Here's how the part is built. I have some questions about the finished solid (model axes, mm). Give positions to 0.01 mm unless a question says otherwise; leave off trailing zeros. Write each loop counter-clockwise with the first axis right and the second up, starting at its lowest first coordinate (ties: lowest second). Pieces come first, ordered by that corner, then holes. Notation, with made-up numbers: (58.25, 14.5) - (86.25, 14.5) arc R10 ccw to (86.25, 33.5) - close; hole circle Ø7 at (-11, -24). An arc over 180 degrees is marked (long way). Write each question's results on one line, items separated by ' | '. Start each with the question number.
Item 1: Suppose I cut it at B-B on z = -24. List the corners of the cut face in (x, y) for me.
Item 2: We'd pull the mould along Z, two halves only. Please class faces 1 (the flat face through (13.496, 1.503, 10.13)), 2 (the flat face through (12.676, 1.503, 60.654)), 3 (the flat face through (2, 3.048, 14)), 4 (the cylindrical face through (-15.875, 1.503, 34.414)): +Z half, -Z half, draft (parallel to the pull), parting line (faces both ways), or undercut.
Item 3: Please list where these lines run through material, in increasing order: line 1 along Z through (x, y) = (-6, 1.7); line 2 along Z through (x, y) = (38, 0.8); line 3 along X through (y, z) = (2.15, -29.5).
Item 4: Will these pins go through, and if not, where does the flat tip stop? P1, Ø1.5, axis at x = 18, y = 1.5, coming from the -Z side; P2, Ø1.5, axis at x = -8.5, y = 2.5, coming from the -Z side; P3, Ø1.5, axis at x = 35, y = 2.5, coming from the +Z side.
Item 5: Suppose I cut it at C-C on x = 35.5. List the corners of the cut face in (y, z) for me, then the cut area to 3 significant figures.
Item 6: Suppose I cut it at A-A on y = 1.1. List the corners of the cut face in (x, z) for me (3 decimals), then the cut area to 3 significant figures.
```python
from build123d import *

# Parameters (mm, degrees)
F0_R     = 3.4358661268
F0_R_2   = 3.175
F1_DEPTH = 3.048


with BuildPart() as f1:
    # F0 (on Front) → F1 (new body)
    with BuildSketch(Plane.XZ):
        with BuildLine():
            ThreePointArc((-9.5183396769, 84.8296558798), (0.1781005018, 75.6624598361), (9.525, 85.1857946098))
            ThreePointArc((9.525, 85.1857946098), (9.5225589236, 85.4014251892), (9.5152369456, 85.6169452446))
            ThreePointArc((9.5152369456, 85.6169452446), (-0.3936477394, 94.7026568268), (-9.5183396769, 84.8296558798))
        make_face()
        with Locations((0, 85.1857946098)):
            Circle(F0_R, mode=Mode.SUBTRACT)
        with BuildLine():
            ThreePointArc((50.9971381625, -29.1142053902), (48.756887413, -23.5666769907), (43.2925762854, -21.1304711977))
            ThreePointArc((43.2925762854, -21.1304711977), (35.0195540586, -29.1142053902), (43.2925762854, -37.0979395828))
            ThreePointArc((43.2925762854, -37.0979395828), (48.756887413, -34.6617337898), (50.9971381625, -29.1142053902))
        make_face()
        with Locations((43.0083461106, -29.1142053902)):
            Circle(F0_R_2, mode=Mode.SUBTRACT)
        with BuildLine():
            ThreePointArc((9.5152369456, 85.6169452446), (9.5225589236, 85.4014251892), (9.525, 85.1857946098))
            ThreePointArc((9.525, 85.1857946098), (0.1781005018, 75.6624598361), (-9.5183396769, 84.8296558798))
            Line((-9.5183396769, 84.8296558798), (-15.7453232111, 36.4107444804))
            ThreePointArc((-15.7453232111, 36.4107444804), (0.0155737272, 50.2607869707), (15.7492659439, 36.3798475748))
            Line((15.7492659439, 36.3798475748), (9.5152369456, 85.6169452446))
        make_face()
        with Locations((-4.955154378, 70.9109946098)):
            Circle(F0_R_2, mode=Mode.SUBTRACT)
        with BuildLine():
            ThreePointArc((9.525, -29.1142053902), (-0.4763850058, -19.6011258506), (-9.477347995, -30.0657830179))
            ThreePointArc((-9.477347995, -30.0657830179), (-6.3899079843, -36.1778235107), (0, -38.6392053902))
            Line((0, -38.6392053902), (0.6773435479, -38.6150911762))
            ThreePointArc((0.6773435479, -38.6150911762), (6.9705567315, -35.6055044785), (9.525, -29.1142053902))
        make_face()
        with Locations((0, -29.1142053902)):
            Circle(F0_R_2, mode=Mode.SUBTRACT)
        with BuildLine():
            ThreePointArc((15.7492659439, 32.3917416448), (0.0155737272, 18.5108022489), (-15.7453232111, 32.3608447391))
            Line((-15.7453232111, 32.3608447391), (-9.477347995, -30.0657830179))
            ThreePointArc((-9.477347995, -30.0657830179), (-0.4763850058, -19.6011258506), (9.525, -29.1142053902))
            ThreePointArc((9.525, -29.1142053902), (6.9705567315, -35.6055044785), (0.6773435479, -38.6150911762))
            Line((0.6773435479, -38.6150911762), (43.2925762854, -37.0979395828))
            ThreePointArc((43.2925762854, -37.0979395828), (35.0195540586, -29.1142053902), (43.2925762854, -21.1304711977))
            Line((43.2925762854, -21.1304711977), (18.9326805356, -20.2632307233))
            ThreePointArc((18.9326805356, -20.2632307233), (13.2237613326, -17.5434154773), (11.3057365986, -11.5176097586))
            Line((11.3057365986, -11.5176097586), (15.7492659439, 32.3917416448))
        make_face()
        with BuildLine():
            ThreePointArc((15.875, 34.3857946098), (15.843535304, 35.3848011513), (15.7492659439, 36.3798475748))
            ThreePointArc((15.7492659439, 36.3798475748), (0.0155737272, 50.2607869707), (-15.7453232111, 36.4107444804))
            ThreePointArc((-15.7453232111, 36.4107444804), (-15.875, 34.3857946098), (-15.7453232111, 32.3608447391))
            ThreePointArc((-15.7453232111, 32.3608447391), (0.0155737272, 18.5108022489), (15.7492659439, 32.3917416448))
            ThreePointArc((15.7492659439, 32.3917416448), (15.843535304, 33.3867880682), (15.875, 34.3857946098))
        make_face()
        with Locations((0, 34.3857946098)):
            Circle(F0_R_2, mode=Mode.SUBTRACT)
        with Locations((-4.955154378, 70.9109946098)):
            Circle(F0_R_2)
        with Locations((0, -29.1142053902)):
            Circle(F0_R_2)
        with Locations((43.0083461106, -29.1142053902)):
            Circle(F0_R_2)
        with BuildLine():
            Line((0.6773435479, -38.6150911762), (0, -38.6392053902))
            ThreePointArc((0, -38.6392053902), (0.3388863295, -38.6331749277), (0.6773435479, -38.6150911762))
        make_face()
        with Locations((0, 85.1857946098)):
            Circle(F0_R)
        with Locations((0, 34.3857946098)):
            Circle(F0_R_2)
    extrude(amount=-F1_DEPTH)


solid = f1.part
```
Checked values:
1) outline: (-10.09, 0) - (49.15, 0) - (49.15, 3.05) - (-10.09, 3.05) - close
2) face 1: undercut | face 2: +Z half | face 3: draft | face 4: parting line
3) line 1: z = -36.51 to 92.58 | line 2: z = -37.29 to -20.94 | line 3: x = -9.53 to 50.99
4) P1: stops at z = -38.03 | P2: stops at z = -34.65 | P3: stops at z = -20.81
5) outline: (0, -37.38) - (3.05, -37.38) - (3.05, -20.85) - (0, -20.85) - close | area: 50.4 mm^2
6) outline: (-15.745, 32.361) - (-9.477, -30.066) arc R9.525 ccw to (0.677, -38.615) - (43.293, -37.098) arc R7.989 ccw to (43.293, -21.13) - (18.933, -20.263) arc R7.95 cw to (11.306, -11.518) - (15.749, 32.392) arc R15.875 ccw to (15.749, 36.38) - (9.515, 85.617) arc R9.525 ccw to (-9.518, 84.83) - (-15.745, 36.411) arc R15.875 ccw to start | area: 3,910 mm^2
